Source: CAD feature listing. Evaluate the final solid. Frame: model axes, mm. Face numbers are marked on the shaded views. A direction names the side the tool comes from. Round coordinates to 2 decimals unless told otherwise and drop trailing zeros. Loops run counter-clockwise (first coordinate to the right, second up) from the corner with the lowest first, then second, coordinate; pieces in that order, holes last. Notation, with made-up numbers: M 5.5,41.25 L 40.5,41.25 A37 ccw 40.5,79.25 Z; hole C -38,-5 d2. An arc over 180 degrees is marked long. Answer as a JSON object with one key per item and string values.
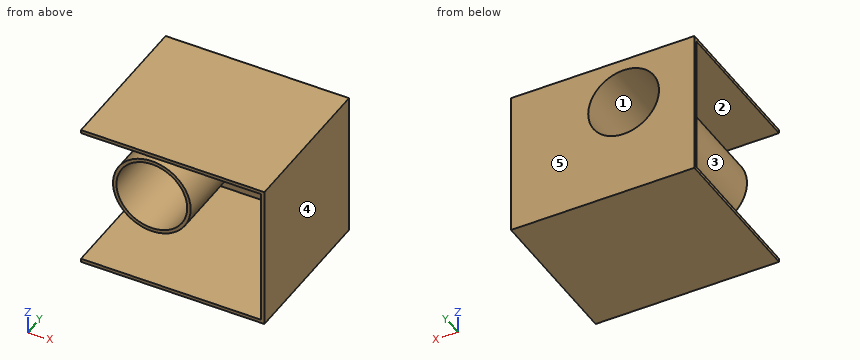
from build123d import *

# Parameters (mm, degrees)
F0_W     = 107.5063981116
F0_H     = 105.9287339449
F0_R     = 25.6439275176
F1_DEPTH = 25.4
F2_DEPTH = 85.598
F3_DEPTH = 25.4
F4_T     = -2.5


with BuildPart() as f1:
    # F0 (on Front) → F1 (new body)
    with BuildSketch(Plane.XZ):
        with Locations((-1.0142084211, -1.1269003153)):
            Rectangle(F0_W, F0_H)
        with Locations((-28.848676011, 18.0304218084)):
            Circle(F0_R, mode=Mode.SUBTRACT)
    extrude(amount=F1_DEPTH)

    # F2 (add): faces of the model
    f2_faces = [f1.faces().sort_by_distance(p)[0] for p in [
        (5.1544323565, -25.4, -5.372522692),
        (5.1544323565, 0, -5.372522692),
    ]]
    extrude(f2_faces, amount=F2_DEPTH, dir=(0, -1, 0))

    # F3 (add): faces of the model
    f3_faces = [f1.faces().sort_by_distance(p)[0] for p in [
        (-54.7674074769, -55.499, -1.1269003153),
        (52.7389906347, -55.499, -1.1269003153),
    ]]
    extrude(f3_faces, amount=F3_DEPTH, dir=(-1, 0, 0))

    # F4
    f4_openings = [f1.faces().sort_by_distance(p)[0] for p in [
        (-11.111372, -110.998, -4.42159),
        (-80.167407, -55.499, -1.1269),
    ]]
    offset(amount=F4_T, openings=f4_openings)


solid = f1.part
Item 1: Section A-A on y = -67. Return the cut outline in (x, z).
Answer sheet:
{"outline": "M -80.17,-54.09 L 52.74,-54.09 L 52.74,51.84 L -80.17,51.84 L -80.17,49.34 L 50.24,49.34 L 50.24,-51.59 L -80.17,-51.59 Z; C -28.85,18.03 d56.29; hole C -28.85,18.03 d51.29"}
Item 2: Line query: probe 1 along Z at (x, y) = (-73, -48); probe 2 along X at (y, z) = (-43, 33); probe 3 along Z at (x, y) = (-21, -40). Output: solid intervals per line, ascending. Write a range as from..to.
Answer sheet:
{"probe 1": "z = -54.09..-51.59, 49.34..51.84", "probe 2": "x = -52.68..-49.67, -8.03..-5.02, 50.24..52.74", "probe 3": "z = -54.09..-51.59, -9..-6.38, 42.44..45.06, 49.34..51.84"}
Item 3: Access query for the marked faces 1 and 2. Directions: +Z, -Z, +X, -X, +Y, -Y. A direction counts if a zero-diameter tool reaches every point of the face in a straight line with its end or side. Return the directions, or none.
Answer sheet:
{"face 1": "+Y, -Y", "face 2": "-X, -Y"}
Item 4: Section C-C on z = 39. Return the cut outline in (x, y), then the cut area to 3 significant figures.
Answer sheet:
{"outline": "M -80.17,-2.5 L -47.62,-2.5 L -47.62,-111 L -43.61,-111 L -43.61,0 L -80.17,0 Z; M -14.09,-111 L -10.08,-111 L -10.08,-2.5 L 50.24,-2.5 L 50.24,-111 L 52.74,-111 L 52.74,0 L -14.09,0 Z", "area": "1,400 mm²"}
Item 5: Pull-direction query (X, two-part tool) for the marked faces 3, 4 and 5; classes: pulls with the +X half, pulls with the -X half, needs draft (parallel to the pull), parting line crosses it, or undercut.
Answer sheet:
{"face 3": "undercut", "face 4": "pulls with the +X half", "face 5": "needs draft"}
Item 6: Contact query for a flat-ended pin moving along its axis: pin 1 Ø4 at (x, z) = (32.5, 10.5) entering from -Y. Output: stop coordinate, or through.
Answer sheet:
{"pin 1": "stops at y = -2.5"}
Item 7: Section B-B on x = 5. Return the cut outline in (y, z).
Answer sheet:
{"outline": "M -111,-54.09 L 0,-54.09 L 0,51.84 L -111,51.84 L -111,49.34 L -2.5,49.34 L -2.5,-51.59 L -111,-51.59 Z"}
Item 8: Section D-D on x = -47.5. Return the cut outline in (y, z), then the cut area to 3 significant figures.
Answer sheet:
{"outline": "M -111,-54.09 L 0,-54.09 L 0,0.43 L -111,0.43 L -111,-3.05 L -2.5,-3.05 L -2.5,-51.59 L -111,-51.59 Z; M -111,35.63 L 0,35.63 L 0,51.84 L -111,51.84 L -111,49.34 L -2.5,49.34 L -2.5,39.11 L -111,39.11 Z", "area": "1,470 mm²"}
